```python
from build123d import *

# Parameters (mm, degrees)
SKETCH1_W           = 125
SKETCH1_H           = 76.2
BOSS_EXTRUDE1_DEPTH = 3
SKETCH2_W           = 3
SKETCH2_H           = 76.2
BOSS_EXTRUDE2_DEPTH = 50
SKETCH4_W           = 53
SKETCH4_H           = 4
BOSS_EXTRUDE4_DEPTH = 21.59
SKETCH5_W           = 53
SKETCH5_H           = 4
BOSS_EXTRUDE5_DEPTH = 21.59
SKETCH6_W           = 168.18
SKETCH6_H           = 25.4
BOSS_EXTRUDE6_DEPTH = 3
CHAMFER1_SIZE       = 28
SKETCH7_W           = 93.6
SKETCH7_H           = 26
CUT_EXTRUDE1_DEPTH  = 2
SKETCH9_W           = 119
SKETCH9_H           = 3
BOSS_EXTRUDE7_DEPTH = 50
CHAMFER2_SIZE       = 4
CHAMFER3_SIZE       = 5
CUT_EXTRUDE2_START  = -0.6
CUT_EXTRUDE2_DEPTH  = 0.6
SKETCH11_R          = 1.75
CUT_EXTRUDE3_DEPTH  = 5
FILLET1_R           = 1
CHAMFER4_SIZE       = 1.5
SKETCH13_R          = 1.75
CUT_EXTRUDE4_DEPTH  = 10


# Read off the part's stored shape, not the designer's step: Cut-Extrude2
with BuildPart() as part:
    # Sketch1 → Boss-Extrude1 (new body)
    with BuildSketch(Plane.XY):
        Rectangle(SKETCH1_W, SKETCH1_H)
    extrude(amount=BOSS_EXTRUDE1_DEPTH)

    # Sketch2 → Boss-Extrude2 (add)
    with BuildSketch(Plane.XY.offset(3)):
        with Locations((-61, 0)):
            Rectangle(SKETCH2_W, SKETCH2_H)
        with Locations((61, 0)):
            Rectangle(SKETCH2_W, SKETCH2_H)
    extrude(amount=BOSS_EXTRUDE2_DEPTH)

    # Sketch4 → Boss-Extrude4 (add)
    with BuildSketch(Plane.ZY.offset(62.5)):
        with Locations((26.5, 36.1)):
            Rectangle(SKETCH4_W, SKETCH4_H)
    extrude(amount=BOSS_EXTRUDE4_DEPTH)

    # Sketch5 → Boss-Extrude5 (add)
    with BuildSketch(Plane(origin=(62.5, 0, 0), x_dir=(0, 0, -1), z_dir=(1, 0, 0))):
        with Locations((-26.5, 36.1)):
            Rectangle(SKETCH5_W, SKETCH5_H)
    extrude(amount=BOSS_EXTRUDE5_DEPTH)

    # Sketch6 → Boss-Extrude6 (add)
    with BuildSketch(Plane(origin=(0, 0, 0), x_dir=(-1, 0, 0), z_dir=(0, 0, -1))):
        with Locations((0, 50.8)):
            Rectangle(SKETCH6_W, SKETCH6_H)
    extrude(amount=-BOSS_EXTRUDE6_DEPTH)

    # Chamfer1
    chamfer1_edges = [part.edges().sort_by_distance(p)[0] for p in [
        (-84.09, 63.5, 1.5),
        (84.09, 63.5, 1.5),
    ]]
    chamfer(chamfer1_edges, length=CHAMFER1_SIZE)

    # Sketch7 → Cut-Extrude1 (cut)
    with BuildSketch(Plane.XY.offset(3)):
        with Locations((0, -9.4)):
            Rectangle(SKETCH7_W, SKETCH7_H)
        with Locations((0, 36.6)):
            Rectangle(SKETCH7_W, SKETCH7_H)
    extrude(amount=-CUT_EXTRUDE1_DEPTH, mode=Mode.SUBTRACT)

    # Sketch9 → Boss-Extrude7 (add)
    with BuildSketch(Plane.XY.offset(3)):
        with Locations((0, -36.6)):
            Rectangle(SKETCH9_W, SKETCH9_H)
    extrude(amount=BOSS_EXTRUDE7_DEPTH)

    # Chamfer2
    chamfer2_edges = [part.edges().sort_by_distance(p)[0] for p in [
        (-59.5, -35.1, 28),
        (59.5, -35.1, 28),
    ]]
    chamfer(chamfer2_edges, length=CHAMFER2_SIZE)

    # Chamfer3
    chamfer3_edges = [part.edges().sort_by_distance(p)[0] for p in [
        (62.5, -38.1, 26.5),
        (-62.5, -38.1, 26.5),
    ]]
    chamfer(chamfer3_edges, length=CHAMFER3_SIZE)

    # Cut-Extrude2 outline → Cut-Extrude2 (cut)
    # profile 1 of 4: a face of its own
    with BuildSketch(Plane.XY.offset(3).offset(CUT_EXTRUDE2_START)):
        with BuildLine():
            Line((-12.843793417, 16.784775128), (-13.918894641, 13.722312614))
            add(Edge.make_bspline(
                [(-13.918894641, 13.722312614), (-13.950745906, 13.608646354), (-13.97919001, 13.483685694), (-14.011317489, 13.235305925), (-14.01541758, 13.110841548), (-13.989547543, 12.867284383), (-13.959604678, 12.747961158), (-13.857332343, 12.519974586), (-13.78490702, 12.411398187), (-13.592313629, 12.212018271), (-13.472083062, 12.121314997), (-13.184369222, 11.962818623), (-13.016909084, 11.895027419), (-12.454211206, 11.728033285), (-11.997806272, 11.664794493), (-11.025815686, 11.62704002), (-10.511530183, 11.651603075), (-9.78258436, 11.770518687), (-9.546683753, 11.824200176), (-9.102156978, 11.962599668), (-8.89364967, 12.047436893), (-8.514064046, 12.246658938), (-8.343153207, 12.361026326), (-8.04132547, 12.611058926), (-7.910418089, 12.746448479), (-7.679883041, 13.0275306), (-7.579636344, 13.172799488), (-7.44297026, 13.39668043), (-7.39971151, 13.472431032), (-7.318663078, 13.627460279), (-7.280772846, 13.706786212), (-7.248185858, 13.788667895)],
                knots=[0, 0, 0, 0, 0.0625, 0.0625, 0.125, 0.125, 0.1875, 0.1875, 0.25, 0.25, 0.3125, 0.3125, 0.375, 0.375, 0.5, 0.5, 0.625, 0.625, 0.6875, 0.6875, 0.75, 0.75, 0.8125, 0.8125, 0.875, 0.875, 0.9375, 0.9375, 0.96875, 0.96875, 1, 1, 1, 1], degree=3))
            Line((-7.248185858, 13.788667895), (-6.196379448, 16.784775128))
            Line((-6.196379448, 16.784775128), (-7.771512854, 16.784775171))
            Line((-7.771512854, 16.784775171), (-8.779640442, 13.913087848))
            add(Edge.make_bspline(
                [(-8.779640442, 13.913087848), (-8.801212863, 13.867686768), (-8.828630281, 13.811426743), (-8.890437912, 13.684919137), (-8.925723343, 13.615289873), (-9.014867696, 13.477778317), (-9.069034752, 13.410065742), (-9.20356673, 13.286811644), (-9.283951715, 13.231246188), (-9.470687062, 13.136081945), (-9.576947425, 13.096402347), (-9.809000897, 13.032201026), (-9.934689567, 13.00760449), (-10.326953956, 12.952228061), (-10.607716868, 12.939250309), (-11.138236784, 12.940792557), (-11.387946526, 12.95495502), (-11.815776289, 13.010911905), (-11.994686961, 13.05312605), (-12.19022456, 13.154353945), (-12.243244201, 13.194586759), (-12.322270156, 13.289978248), (-12.348136332, 13.345299657), (-12.373130151, 13.46826163), (-12.371956966, 13.5361378), (-12.35254935, 13.67085438), (-12.333771283, 13.737944141), (-12.322165603, 13.788667937)],
                knots=[0, 0, 0, 0, 0.0625, 0.0625, 0.125, 0.125, 0.1875, 0.1875, 0.25, 0.25, 0.3125, 0.3125, 0.375, 0.375, 0.5, 0.5, 0.625, 0.625, 0.75, 0.75, 0.8125, 0.8125, 0.875, 0.875, 0.9375, 0.9375, 1, 1, 1, 1], degree=3))
            Line((-12.322165603, 13.788667937), (-11.2703582, 16.784775128))
            Line((-11.2703582, 16.784775128), (-12.843793417, 16.784775128))
        make_face()
    # profile 2 of 4: a face of its own
    with BuildSketch(Plane.XY.offset(3).offset(CUT_EXTRUDE2_START)):
        Polygon((14.082145905, 15.466432145), (14.547318434, 16.784775128), (8.481425261, 16.784775128), (8.015662645, 15.45803385), (10.386127447, 15.45803385), (9.075451111, 11.743439605), (10.661733364, 11.743439605), (11.975372051, 15.466432145), align=None)
    # profile 3 of 4: a face of its own
    with BuildSketch(Plane.XY.offset(3).offset(CUT_EXTRUDE2_START)):
        Polygon((0.359928822, 15.45803385), (0.825593089, 16.784775128), (-5.237786258, 16.784775128), (-5.705919648, 15.45803385), (-3.328357423, 15.45803385), (-4.639000977, 11.723834147), (-3.059652234, 11.723834147), (-1.74900868, 15.45803385), align=None)
    # profile 4 of 4: a face of its own
    with BuildSketch(Plane.XY.offset(3).offset(CUT_EXTRUDE2_START)):
        Polygon((7.732615088, 18.009820452), (8.67993853, 22.298690548), (4.451236342, 18.010625114), (-13.617285872, 18.010625114), (-13.760696138, 17.631800344), (4.083976363, 17.631800344), (-2.561139847, 10.89339914), (-16.036862666, 10.89339914), (-16.175076152, 10.505618026), (-2.943552817, 10.505618026), (-8.264964605, 5.10950355), (-0.819885517, 10.505618026), (5.569839691, 10.505618026), (5.813932632, 9.32327198), (6.07620201, 10.510665049), (13.482070183, 10.510665049), (13.624063348, 10.89339914), (6.160742258, 10.89339914), (7.649117922, 17.631800344), (15.972876762, 17.631800344), (16.113123511, 18.009820452), align=None)
        Polygon((-0.283933962, 10.894070437), (4.780674194, 14.564845582), (5.489286994, 10.894070437), align=None, mode=Mode.SUBTRACT)
        Polygon((5.863139247, 17.323666682), (5.364033793, 14.945937564), (5.179256414, 15.9244998), (2.885975157, 14.289472868), align=None, mode=Mode.SUBTRACT)
    extrude(amount=CUT_EXTRUDE2_DEPTH, mode=Mode.SUBTRACT)

    # Sketch11 → Cut-Extrude3 (cut)
    with BuildSketch(Plane(origin=(0, 38.1, 0), x_dir=(1, 0, 0), z_dir=(0, 1, 0))):
        with Locations(Location((-76.11, -13, 0), (0, 0, 270))):
            Circle(SKETCH11_R)
        with Locations(Location((76.29, -13, 0), (0, 0, 270))):
            Circle(SKETCH11_R)
    extrude(amount=-CUT_EXTRUDE3_DEPTH, mode=Mode.SUBTRACT)

    # Fillet1
    fillet1_edges = [part.edges().sort_by_distance(p)[0] for p in [
        (-62.5, 34.1, 26.5),
        (62.5, 34.1, 26.5),
    ]]
    fillet(fillet1_edges, radius=FILLET1_R)

    # Chamfer4
    chamfer4_edges = [part.edges().sort_by_distance(p)[0] for p in [
        (-59.5, 38.1, 28),
        (59.5, 38.1, 28),
    ]]
    chamfer(chamfer4_edges, length=CHAMFER4_SIZE)

    # Sketch13 → Cut-Extrude4 (cut)
    with BuildSketch(Plane(origin=(0, 38.1, 0), x_dir=(1, 0, 0), z_dir=(0, 1, 0))):
        with Locations(Location((-76.29, -38.4, 0), (0, 0, 270))):
            Circle(SKETCH13_R)
        with Locations(Location((76.11, -38.4, 0), (0, 0, 270))):
            Circle(SKETCH13_R)
    extrude(amount=-CUT_EXTRUDE4_DEPTH, mode=Mode.SUBTRACT)


solid = part.part
```
Geometry check sheet. Reference: the model listing, model coordinates, mm. A direction names the side the tool comes from. Give positions to 0.01 mm unless a question says otherwise; leave off trailing zeros. Loops run counter-clockwise (first coordinate to the right, second up) from the corner with the lowest first, then second, coordinate; pieces in that order, holes last. Notation, with made-up numbers: M 28,18.5 L 40,18.5 A29 cw 40,54.5 Z; hole C 22.25,67.5 d3. An arc over 180 degrees is marked long. Answer as CSV lines item,"result".
Item 1: Cross-section at C-C on y = -14. Record the cut outline in (x, z), and give its area (3 significant figures).
Values:
outline,"M -62.5,0 L 62.5,0 L 62.5,53 L 59.5,53 L 59.5,3 L 46.8,3 L 46.8,1 L -46.8,1 L -46.8,3 L -59.5,3 L -59.5,53 L -62.5,53 Z"
area,"488 mm²"
Item 2: Cross-section at D-D on y = -28. Record the cut outline in (x, z).
Values:
outline,"M -62.5,0 L 62.5,0 L 62.5,53 L 59.5,53 L 59.5,3 L -59.5,3 L -59.5,53 L -62.5,53 Z"
Item 3: Access from +Z, -Z, +X, -X, +Y, -Y to the whole of each face (thin tool, end or side, straight path). Record for faces 4 (the flat face through (-1, -35.1, 28)), 5 (the flat face through (62.5, 0, 26)), 6 (the flat face through (-1, -9, 1)).
Values:
face 4,"+Z, +Y"
face 5,"+Z, -Z, +X, -Y"
face 6,"+Z"
Item 4: Cross-section at B-B on z = 45.5. Record the cut outline in (x, y), and give its area (3 significant figures).
Values:
outline,"M -84.09,34.1 L -63.5,34.1 A1 cw -62.5,33.1 L -62.5,-33.1 L -57.5,-38.1 L 57.5,-38.1 L 62.5,-33.1 L 62.5,33.1 A1 cw 63.5,34.1 L 84.09,34.1 L 84.09,35.5 L 81.49,38.1 L 61,38.1 L 59.5,36.6 L 59.5,-31.1 L 55.5,-35.1 L -55.5,-35.1 L -59.5,-31.1 L -59.5,36.6 L -61,38.1 L -81.49,38.1 L -84.09,35.5 Z"
area,"969 mm²"
Item 5: Release check for a two-part mould opening along Y. For faces 1 (the flat face through (-82.47, 37.12, 14.6)), 2 (the flat face through (-74, 34.1, 26)), 3 (the flat face through (-1, 37, 1)) record: pulls with the +Y half, pulls with the -Y half, needs draft (parallel to the pull), parting line crosses it, or undercut.
Values:
face 1,"pulls with the +Y half"
face 2,"pulls with the -Y half"
face 3,"undercut"
Item 6: Material ranges on line 1 (Z direction, x = -76.29, y = 35.9); line 2 (X direction, y = -27, z = 7); line 3 (X direction, y = 36.9, z = 38.4), recorded low to high.
Values:
line 1,"z = 0 to 11.26, 14.74 to 36.65, 40.15 to 53"
line 2,"x = -62.5 to -59.5, 59.5 to 62.5"
line 3,"x = -82.69 to -78.04, -74.54 to -59.8, 59.8 to 74.36, 77.86 to 82.69"
Item 7: Cross-section at A-A on z = 13. Count the separate pieces of the cut face and the enclosed holes in it, and give its area (3 significant figures).
Values:
separate pieces,"3"
enclosed holes,"0"
area,"941 mm²"
Item 8: Depth check by flat-ended pin: P1, Ø8, axis at x = -21.5, y = 37.5, coming from the +Z side; P2, Ø6, axis at y = -10.5, z = 32.5, coming from the +X side; P3, Ø4, axis at x = -57, y = 42.5, coming from the +Z side. Enter the tip coordinate at first touch or a pass-through.
Values:
P1,"stops at z = 1"
P2,"stops at x = 62.5"
P3,"stops at z = 3"
